from build123d import *

# Parameters (mm, degrees)
F0_W     = 98.3996
F0_H     = 149.2123
F1_DEPTH = 1.6002
F2_DEPTH = 50.8
F3_R     = 12.7
F4_DEPTH = 1.6002


with BuildPart() as f1:
    # F0 (on Right) → F1 (new body)
    with BuildSketch(Plane.YZ):
        Polygon((50.8, 76.2), (0, 76.2), (-50.8, 76.2), (-50.8, 0), (-50.8, -76.2), (0, -76.2), (50.8, -76.2), (50.8, 0), align=None)
        with Locations((0, 0.00635)):
            Rectangle(F0_W, F0_H, mode=Mode.SUBTRACT)
        with Locations((0, 0.00635)):
            Rectangle(F0_W, F0_H)
    extrude(amount=-F1_DEPTH)

    # F0 (on Right) → F2 (join)
    with BuildSketch(Plane.YZ):
        Polygon((50.8, 76.2), (0, 76.2), (-50.8, 76.2), (-50.8, 0), (-50.8, -76.2), (0, -76.2), (50.8, -76.2), (50.8, 0), align=None)
        with Locations((0, 0.00635)):
            Rectangle(F0_W, F0_H, mode=Mode.SUBTRACT)
    extrude(amount=F2_DEPTH)

    # F3 (on face) → F4 (cut)
    with BuildSketch(Plane.YZ):
        with Locations((0, 38.1)):
            Circle(F3_R)
        with Locations((0, -50.8)):
            Circle(F3_R)
    extrude(amount=-F4_DEPTH, mode=Mode.SUBTRACT)


solid = f1.part
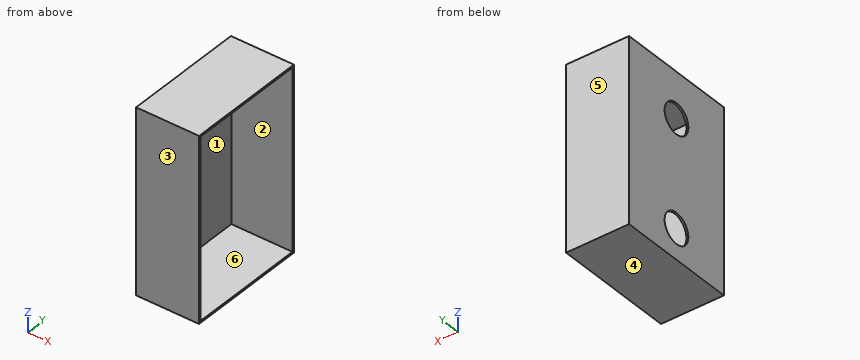
Part model, mm, in its own coordinate system. Face numbers are marked on the shaded views. A direction names the side the tool comes from. Coordinates: 2 decimals unless noted, no trailing zeros. Order: outer loops, then holes, each group sorted by start corner. A loop starts at its lowest first (then second) coordinate and runs counter-clockwise, first axis right, second up. Notation, with made-up numbers: M 0,11 L 51,11 A20 ccw 51,29 Z; hole C 60.5,5.5 d5. An arc over 180 degrees is marked long. Use a Markdown table: item, result.
(1) Tool access for the marked faces 5 and 6: list every direction of +Z, -Z, +X, -X, +Y, -Y with a clear straight run to the whole face (end or side of a thin tool).
A:
| item | result |
|---|---|
| face 5 | +Z, -Z, +X, -X, +Y |
| face 6 | +X |
(2) Flat gauge pin, fed straight in: pin 1 (8 mm diameter, centred on y = 24, z = -7, fed in from +X). Where does the tip first touch, or does it go through?
A:
| item | result |
|---|---|
| pin 1 | stops at x = 0 |
(3) Cut at D-D on y = -41. Write the cut outline in (x, z), then the cut area to 3 significant figures.
A:
| item | result |
|---|---|
| outline | M -1.6,-76.2 L 50.8,-76.2 L 50.8,-74.6 L 0,-74.6 L 0,74.61 L 50.8,74.61 L 50.8,76.2 L -1.6,76.2 Z |
| area | 406 mm^2 |
(4) Cut at A-A on z = 38.1. Write the cut outline in (x, y).
A:
| item | result |
|---|---|
| outline | M -1.6,-50.8 L 50.8,-50.8 L 50.8,-49.2 L 0,-49.2 L 0,-12.7 L -1.6,-12.7 Z; M -1.6,12.7 L 0,12.7 L 0,49.2 L 50.8,49.2 L 50.8,50.8 L -1.6,50.8 Z |
(5) Cut at B-B on y = 0. Write the cut outline in (x, z).
A:
| item | result |
|---|---|
| outline | M -1.6,-76.2 L 50.8,-76.2 L 50.8,-74.6 L 0,-74.6 L 0,-63.5 L -1.6,-63.5 Z; M -1.6,-38.1 L 0,-38.1 L 0,25.4 L -1.6,25.4 Z; M -1.6,50.8 L 0,50.8 L 0,74.61 L 50.8,74.61 L 50.8,76.2 L -1.6,76.2 Z |
(6) Cut at C-C on x = 42.5. Write the cut outline in (y, z).
A:
| item | result |
|---|---|
| outline | M -50.8,-76.2 L 50.8,-76.2 L 50.8,76.2 L -50.8,76.2 Z; hole M -49.2,-74.6 L 49.2,-74.6 L 49.2,74.61 L -49.2,74.61 Z |
(7) Probe L1, parallel to Z at x = -1.2, y = 0; L2, parallel to Y at x = 1.5, z = 46.5; L3, parallel to Z at x = 28.5, y = 3. List the from-to ranges inside material, lowest first.
A:
| item | result |
|---|---|
| L1 | z = -76.2 to -63.5, -38.1 to 25.4, 50.8 to 76.2 |
| L2 | y = -50.8 to -49.2, 49.2 to 50.8 |
| L3 | z = -76.2 to -74.6, 74.61 to 76.2 |
(8) Pull direction Y, two halves, no side cores. Call the marked faces 1, 2, 3 and 4: released by +Y, released by -Y, zero draft, split by the parting line, or undercut.
A:
| item | result |
|---|---|
| face 1 | undercut |
| face 2 | undercut |
| face 3 | released by -Y |
| face 4 | zero draft |
